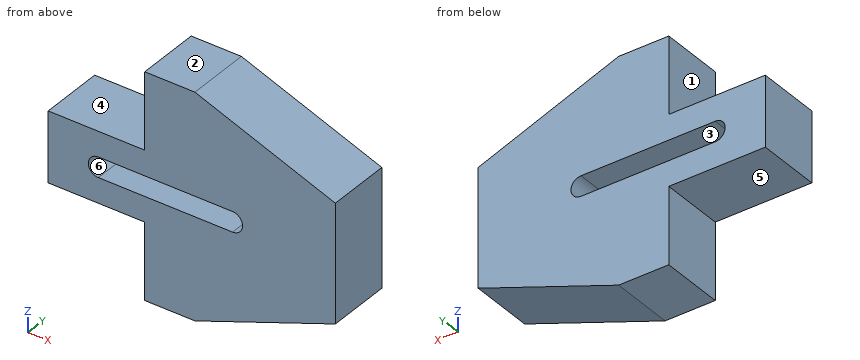
```python
from build123d import *

# Parameters (mm, degrees)
BOSS_EXTRUDE1_DEPTH = 2.55
CUT_EXTRUDE1_DEPTH  = 26.092429137


with BuildPart() as part:
    # Sketch1 → Boss-Extrude1 (new, symmetric)
    with BuildSketch(Plane(origin=(0, 0, 0), x_dir=(1, 0, 0), z_dir=(0, 1, 0))):
        Polygon((-22.9, 0), (-22.9, 2.8), (-15.2, 2.8), (-15.2, 8.9), (-11.2, 8.9), (0, 4.7), (0, 0), align=None)
    boss_extrude1 = extrude(amount=BOSS_EXTRUDE1_DEPTH, both=True)

    # Mirror1: Boss-Extrude1 across plane
    add(boss_extrude1.mirror(Plane.XY))

    # Sketch2 → Cut-Extrude1 (cut, through all)
    with BuildSketch(Plane(origin=(0, 2.55, 0), x_dir=(1, 0, 0), z_dir=(0, 1, 0))):
        with BuildLine():
            Line((-18.9, 0.8), (-8.2, 0.8))
            ThreePointArc((-8.2, 0.8), (-7.4, 0), (-8.2, -0.8))
            Line((-8.2, -0.8), (-18.9, -0.8))
            ThreePointArc((-18.9, -0.8), (-19.7, 0), (-18.9, 0.8))
        make_face()
    extrude(amount=-CUT_EXTRUDE1_DEPTH, mode=Mode.SUBTRACT)


solid = part.part
```
Design review of the part built by this model. Coordinates are the model's own, in mm. Face numbers are marked on the shaded views. A direction names the side the tool comes from. Coordinates: 2 decimals unless noted, no trailing zeros. Order: outer loops, then holes, each group sorted by start corner. A loop starts at its lowest first (then second) coordinate and runs counter-clockwise, first axis right, second up. Notation, with made-up numbers: (4.5, 34.5) - (51.5, 34.5) arc R20 cw to (51.5, 61.5) - close; hole circle Ø8 at (-6, 36.25). An arc over 180 degrees is marked (long way). One line per question, with ' | ' between items.
Q1. Consider section D-D, the plane z = 5. Give the boundary of the cut face in (x, y).
Answer key:
outline: (-15.2, -2.55) - (-0.8, -2.55) - (-0.8, 2.55) - (-15.2, 2.55) - close
Q2. Consider section B-B, the plane z = 0. Give the boundary of the cut face in (x, y).
Answer key:
outline: (-22.9, -2.55) - (-19.7, -2.55) - (-19.7, 2.55) - (-22.9, 2.55) - close; (-7.4, -2.55) - (0, -2.55) - (0, 2.55) - (-7.4, 2.55) - close
Q3. The part is to be moulded in two halves that separate along X. For the marked faces 1, 2 and 3, say which applies: +X half, -X half, draft (parallel to the pull), parting line (faces both ways), or undercut.
Answer key:
face 1: -X half | face 2: draft | face 3: undercut
Q4. Consider section A-A, the plane x = -14.5. Give the boundary of the cut face in (y, z), then the cut area to 3 significant figures.
Answer key:
outline: (-2.55, -8.9) - (2.55, -8.9) - (2.55, -0.8) - (-2.55, -0.8) - close; (-2.55, 0.8) - (2.55, 0.8) - (2.55, 8.9) - (-2.55, 8.9) - close | area: 82.6 mm2
Q5. For the marked faces 4, 5 and 6, list the 3-axis set-ups (+Z, -Z, +X, -X, +Y, -Y) from which the entire face can be reached by the end or side of a thin tool; tool diameter is ignored.
Answer key:
face 4: +Z, -X, +Y, -Y | face 5: -Z, -X, +Y, -Y | face 6: +Y, -Y
Q6. Consider section C-C, the plane y = 2.1. Give the boundary of the cut face in (x, z).
Answer key:
outline: (-22.9, -2.8) - (-15.2, -2.8) - (-15.2, -8.9) - (-11.2, -8.9) - (0, -4.7) - (0, 4.7) - (-11.2, 8.9) - (-15.2, 8.9) - (-15.2, 2.8) - (-22.9, 2.8) - close; hole (-18.9, -0.8) - (-8.2, -0.8) arc R0.8 ccw to (-8.2, 0.8) - (-18.9, 0.8) arc R0.8 ccw to start
Q7. To check wall thickness, follow line 1 along Z through (x, y) = (-19, -1.6); line 2 along Z through (x, y) = (-14.75, 0.25); line 3 along X through (y, z) = (-0.3, -4.5). State the ranges of each line that lie inside material, in increasing order.
Answer key:
line 1: z = -2.8 to -0.79, 0.79 to 2.8 | line 2: z = -8.9 to -0.8, 0.8 to 8.9 | line 3: x = -15.2 to 0
Q8. Clearance check with a flat-ended pin moving along its axis: pin 1 Ø1.5 at (y, z) = (0, -7) entering from -X. State where the tip first meets the part, or that it passes through.
Answer key:
pin 1: stops at x = -15.2
